Geometry check sheet. Reference: the model listing, model coordinates, mm. Face numbers are marked on the shaded views. A direction names the side the tool comes from. Coordinates: 2 decimals unless noted, no trailing zeros. Loops run counter-clockwise (first coordinate to the right, second up) from the corner with the lowest first, then second, coordinate; pieces in that order, holes last.
Autodesk Inventor part; units mm, degrees
ref_plane "YZ Plane" through (0, 0, 0) normal (1, 0, 0) x (0, 1, 0)
ref_plane "XZ Plane" through (0, 0, 0) normal (0, 1, 0) x (-1, 0, 0)
ref_plane "XY Plane" through (0, 0, 0) normal (0, 0, 1) x (1, 0, 0)
sketch "Skizze1" plane through (0, 0, 0) normal (0, 0, 1) x (1, 0, 0)
  line L0 (-30, 0) -> (30, 0)
  line L1 (30, 0) -> (30, -34.5)
  line L2 (30, -34.5) -> (-30, -34.5)
  line L3 (-30, -34.5) -> (-30, 0)
  line L4 (-9.8, 0) -> (9.8, 0)
  line L5 (9.8, 0) -> (9.8, 3.6)
  line L6 (9.8, 3.6) -> (-9.8, 3.6)
  line L7 (-9.8, 3.6) -> (-9.8, 0)
  line L8 (9.8, 3.6) -> (11.4, 3.6)
  line L9 (11.4, 3.6) -> (11.4, 2)
  line L10 (11.4, 2) -> (9.8, 2)
  line L11 (9.8, 2) -> (9.8, 3.6)
  line L12 (-9.8, 3.6) -> (-11.4, 3.6)
  line L13 (-11.4, 3.6) -> (-11.4, 2)
  line L14 (-11.4, 2) -> (-9.8, 2)
  line L15 (-9.8, 2) -> (-9.8, 3.6)
  point P0 (0, 0)
  point P1 (0, 0)
  point P2 (9.8, 1.8)
  dimension "d0" = 3.6
  dimension "d1" = 19.6
  dimension "d2" = 1.6
  dimension "d3" = 1.6
  dimension "d4" = 1.6
  dimension "d5" = 1.6
  dimension "d6" = 34.5
  dimension "d7" = 60
  dimension "d8" = 30
  dimension "d9" = 9.8
extrude "Extrusion1" add sketch "Skizze1" against normal blind 2
sketch "Skizze2" plane through (0, 0, -2) normal (0, 0, -1) x (-1, 0, 0)
  line L0 (-30, -34.5) -> (30, -34.5)
  line L1 (30, -34.5) -> (30, 0)
  line L2 (-30, -34.5) -> (30, -34.5)
  line L3 (30, -34.5) -> (30, -30.5)
  line L4 (30, -30.5) -> (-30, -30.5)
  line L5 (-30, -30.5) -> (-30, -34.5)
  point P0 (0, 0)
  dimension "d12" = 4
extrude "Extrusion2" add sketch "Skizze2" along normal blind 9
sketch "Skizze3" plane through (-30, -34.5, 0) normal (-1, 0, 0) x (0, 0, 1)
  line L0 (-2, 4) -> (-11, 4)
  line L1 (-8.9, 4) -> (-7, 4)
  line L2 (-7, 4) -> (-7, 2)
  line L3 (-7, 2) -> (-8.9, 2)
  line L4 (-8.9, 2) -> (-8.9, 4)
  line L5 (-2, 4) -> (-2, 34.5)
  point P0 (0, 34.5)
  dimension "d15" = 1.9
  dimension "d16" = 2
  dimension "d17" = 5
extrude "Extrusion3" cut sketch "Skizze3" against normal through all
sketch "Skizze4" plane through (-30, -30.5, -2) normal (0, 1, 0) x (1, 0, 0)
  line L0 (60, 0) -> (0, 0)
  line L1 (0, 0) -> (4, 0)
  line L2 (4, 0) -> (4, 4)
  line L3 (4, 4) -> (0, 4)
  line L4 (0, 4) -> (0, 0)
  line L5 (60, -2) -> (60, 9)
  line L6 (60, 0) -> (56, 0)
  line L7 (56, 0) -> (56, 4)
  line L8 (56, 4) -> (60, 4)
  line L9 (60, 4) -> (60, 0)
  point P0 (30, -2)
  point P1 (60, 4)
  point P2 (4, 0)
  dimension "d20" = 4
  dimension "d21" = 4
  dimension "d22" = 4
  dimension "d23" = 4
extrude "Extrusion4" cut sketch "Skizze4" against normal blind 10
sketch "Skizze5" plane through (0, 0, -2) normal (0, 0, -1) x (-1, 0, 0)
  line L0 (30, 0) -> (30, -34.5)
  line L1 (30, -5) -> (15, -5)
  line L2 (15, -5) -> (15, -30)
  line L3 (15, -30) -> (30, -30)
  line L4 (30, -30) -> (30, -5)
  line L5 (30, 0) -> (9.8, 0)
  point P0 (0, 0)
  point P1 (30, -30.5)
  dimension "d28" = 15
  dimension "d29" = 25
  dimension "d30" = 5
extrude "Extrusion5" cut sketch "Skizze5" against normal blind 10
equation "\"d2\" = d4"
equation "\"d3\" = d4"
equation "\"d5\" = d4"
properties part number "ClipUnten"
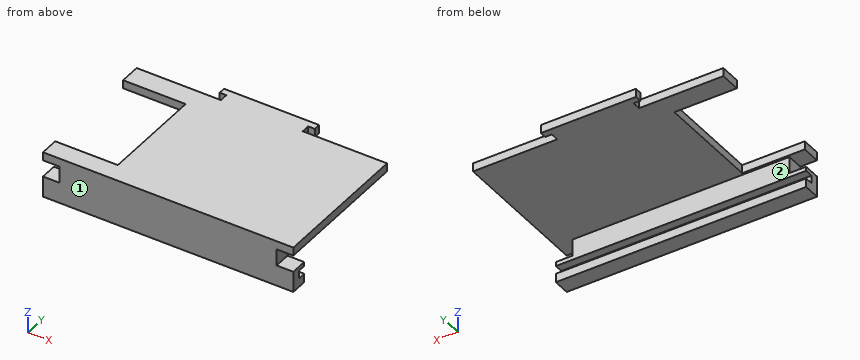
(1) Scan lines: L1, parallel to Z at x = 18, y = -32; L2, parallel to Y at x = -17, z = -1; L3, parallel to Y at x = -18, z = -6.5. Record each from-to range of solid material in increasing order.
Findings:
L1: z = -11 to -8.9, -7 to 0
L2: y = -34.5 to -30, -5 to 0
L3: y = -34.5 to -30.5
(2) Access from +Z, -Z, +X, -X, +Y, -Y to the whole of each face (thin tool, end or side, straight path). Record for the marked faces 1 and 2.
Findings:
face 1: +Z, -Z, +X, -X, -Y
face 2: -Z, +X, -X, +Y
(3) Sectioned sample at C-C on z = -8.25. Record the cut outline in (x, y).
Findings:
outline: (-30, -34.5) - (30, -34.5) - (30, -32.5) - (-30, -32.5) - close
(4) Sectioned sample at A-A on x = -20.5. Record the cut outline in (y, z).
Findings:
outline: (-34.5, -11) - (-30.5, -11) - (-30.5, -8.9) - (-32.5, -8.9) - (-32.5, -7) - (-30.5, -7) - (-30.5, -2) - (-30, -2) - (-30, 0) - (-34.5, 0) - close; (-5, -2) - (0, -2) - (0, 0) - (-5, 0) - close
(5) Sectioned sample at B-B on x = 16. Record the cut outline in (y, z), and give its area (3 significant figures).
Findings:
outline: (-34.5, -11) - (-30.5, -11) - (-30.5, -8.9) - (-32.5, -8.9) - (-32.5, -7) - (-30.5, -7) - (-30.5, -2) - (0, -2) - (0, 0) - (-34.5, 0) - close
area: 101 mm2
(6) Gauge pin test, flat ends, axial feed: pin 1 Ø1.2 at (y, z) = (-32.5, -3.5) entering from -X; pin 2 Ø1 at (y, z) = (-20, -0.5) entering from -X; pin 3 Ø1.5 at (x, z) = (11.5, -5.5) entering from +Y. Record the tip position at first contact, or that the pin passes through.
Findings:
pin 1: stops at x = -26
pin 2: stops at x = -15
pin 3: stops at y = -30.5
(7) Sectioned sample at D-D on y = -17.5. Record the cut outline in (x, z).
Findings:
outline: (-15, -2) - (30, -2) - (30, 0) - (-15, 0) - close
